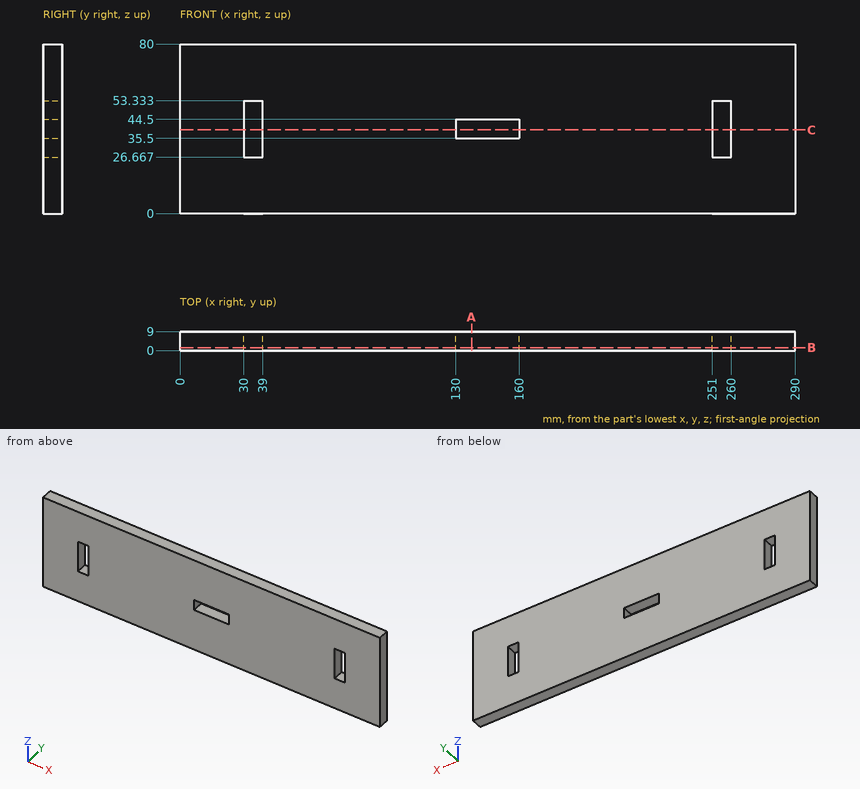
Geometry check sheet. Reference: drawing and pictorial views, mm from the part's lowest x, y, z. Give positions to 0.01 mm unless a question says otherwise; leave off trailing zeros. Order: outer loops, then holes, each group sorted by start corner. A loop starts at its lowest first (then second) coordinate and runs counter-clockwise, first axis right, second up. Notation, with made-up numbers: M 35.25,-38 L 87.25,-38 A8 ccw 87.25,-34 Z; hole C 71.25,3.5 d7. An arc over 180 degrees is marked long. Return JSON: item names as keys, results as strings. Group by question number.
1) Section check C-C on z = 39.5. Record the cut outline in (x, y), and give its area (3 significant figures).
2) Section check A-A on x = 137.5. Record the cut outline in (y, z), and give its area (3 significant figures).
3) Section check B-B on y = 1.5. Record the cut outline in (x, z), and give its area (4 significant figures).
4) Scan lines: line 1 (X direction, y = 3.5, z = 46); line 2 (Z direction, x = 154, y = 0.5). Record each from-to range of solid material in increasing order.
Answer block:
{
 "1": {"outline": "M 0,0 L 30,0 L 30,9 L 0,9 Z; M 39,0 L 130,0 L 130,9 L 39,9 Z; M 160,0 L 251,0 L 251,9 L 160,9 Z; M 260,0 L 290,0 L 290,9 L 260,9 Z", "area": "2,180 mm^2"},
 "2": {"outline": "M 0,0 L 9,0 L 9,35.5 L 0,35.5 Z; M 0,44.5 L 9,44.5 L 9,80 L 0,80 Z", "area": "639 mm^2"},
 "3": {"outline": "M 0,0 L 290,0 L 290,80 L 0,80 Z; hole M 30,26.67 L 39,26.67 L 39,53.33 L 30,53.33 Z; hole M 130,35.5 L 160,35.5 L 160,44.5 L 130,44.5 Z; hole M 251,26.67 L 260,26.67 L 260,53.33 L 251,53.33 Z", "area": "22,450 mm^2"},
 "4": {"line 1": "x = 0 to 30, 39 to 251, 260 to 290", "line 2": "z = 0 to 35.5, 44.5 to 80"}
}
